Geometry: final body of the model. Coordinates: model frame, mm. A direction names the side the tool comes from. Round coordinates to 2 decimals unless told otherwise and drop trailing zeros. Loops run counter-clockwise (first coordinate to the right, second up) from the corner with the lowest first, then second, coordinate; pieces in that order, holes last. Notation, with made-up numbers: (-32.75, -10) - (-14.75, -10) arc R19 ccw to (-14.75, 13) - close; hole circle Ø11 at (-21, 42). An arc over 180 degrees is marked (long way). Answer as a JSON object with one key per item and string values. Group by question number.
Item 1: Section C-C (z = 24.5). Count the separate pieces of the cut face and the enclosed holes in it, plus the area to 3 significant figures.
Item 2: Section D-D (x = 21). Return the cut outline in (y, z), plus the area to 3 significant figures.
Item 3: Section A-A (z = 7). Return the cut outline in (x, y).
Item 4: Reachability of faces 4 (the face through (37, 65, 5.25)), 5 (the face through (69, 75, 15)) from +Z, -Z, +X, -X, +Y, -Y: full face, straight path, thin tool, end or side. Return the list, or none.
Item 5: First-contact query: pin 1 (17.5 mm diameter, centred on x = 108.5, y = 36, fed in from +Z); pin 2 (1.7 mm diameter, centred on x = 129.5, y = 67, fed in from +Z); pin 3 (6 mm diameter, centred on x = 19, y = 33.5, fed in from +Z). Flat tips, straight axial feed; report the tip coordinate or a pass-through.
Item 6: Line query: line 1 (X direction, y = 37.5, z = 2.15); line 2 (Y direction, x = 105, z = 12.75); line 3 (Y direction, x = 106, z = 27.5). Output: solid intervals per line, ascending.
Item 7: Draft query along X for faces 1 (the face through (140, 37, 15)), 2 (the face through (69, 0, 15)), 3 (the face through (130, 8, 10)). Return one class per face: released by +X, released by -X, zero draft, split by the parting line, or undercut.
Item 8: Section B-B (x = 105). Return the cut outline in (y, z), plus the area to 3 significant figures.
```python
from build123d import *

# Parameters (mm, degrees)
ESQUISSE1_W                  = 140
ESQUISSE1_H                  = 75
BOSS_EXTRU_1_DEPTH           = 30
ESQUISSE2_R                  = 31
ENL_V_MAT_EXTRU_1_DEPTH      = 25
ENL_V_MAT_EXTRU_2_DEPTH      = 161.779351908
ENL_V_MAT_EXTRU_2_DEPTH_BACK = 161.779351908
ESQUISSE3_R                  = 3.4
BOSS_EXTRU_2_START           = 0.25
ESQUISSE4_R                  = 31
ESQUISSE4_R_2                = 27.01
BOSS_EXTRU_2_DEPTH           = 0.25
BOSS_EXTRU_3_START           = 7.9
ESQUISSE5_R                  = 7.99
ESQUISSE5_R_2                = 3.4
BOSS_EXTRU_3_DEPTH           = 7.9
ESQUISSE6_R                  = 1.65
ENL_V_MAT_EXTRU_3_DEPTH      = 20


with BuildPart() as part:
    # Esquisse1 → Boss.-Extru.1 (new body)
    with BuildSketch(Plane.XY):
        with Locations((70, 37.5)):
            Rectangle(ESQUISSE1_W, ESQUISSE1_H)
    extrude(amount=BOSS_EXTRU_1_DEPTH)

    # Esquisse2 → Enlèv. mat.-Extru.1 (cut)
    with BuildSketch(Plane.XY.offset(30)):
        with Locations((35, 37.5)):
            Circle(ESQUISSE2_R)
        with Locations(Location((105, 37.5, 0), (0, 0, 180))):
            Circle(ESQUISSE2_R)
    extrude(amount=-ENL_V_MAT_EXTRU_1_DEPTH, mode=Mode.SUBTRACT)

    # Esquisse3 → Enlèv. mat.-Extru.2 (cut, two sides: drawn at the far end of the back side and taken through both)
    with BuildSketch(Plane.XY.offset(5).offset(-ENL_V_MAT_EXTRU_2_DEPTH_BACK)):
        with Locations((35, 37.5)):
            Circle(ESQUISSE3_R)
        with Locations(Location((105, 37.5, 0), (0, 0, 180))):
            Circle(ESQUISSE3_R)
    extrude(amount=ENL_V_MAT_EXTRU_2_DEPTH + ENL_V_MAT_EXTRU_2_DEPTH_BACK, mode=Mode.SUBTRACT)

    # Esquisse4 → Boss.-Extru.2 (add)
    # profile 1 of 2: a face of its own
    with BuildSketch(Plane.XY.offset(5).offset(BOSS_EXTRU_2_START)):
        with Locations((35, 37.5)):
            Circle(ESQUISSE4_R)
        with Locations((35, 37.5)):
            Circle(ESQUISSE4_R_2, mode=Mode.SUBTRACT)
    # profile 2 of 2: a face of its own
    with BuildSketch(Plane.XY.offset(5).offset(BOSS_EXTRU_2_START)):
        with Locations(Location((105, 37.5, 0), (0, 0, 180))):
            Circle(ESQUISSE4_R)
        with Locations(Location((105, 37.5, 0), (0, 0, 180))):
            Circle(ESQUISSE4_R_2, mode=Mode.SUBTRACT)
    extrude(amount=-BOSS_EXTRU_2_DEPTH)

    # Esquisse5 → Boss.-Extru.3 (add)
    # profile 1 of 2: a face of its own
    with BuildSketch(Plane.XY.offset(5).offset(BOSS_EXTRU_3_START)):
        with Locations((35, 37.5)):
            Circle(ESQUISSE5_R)
        with Locations((35, 37.5)):
            Circle(ESQUISSE5_R_2, mode=Mode.SUBTRACT)
    # profile 2 of 2: a face of its own
    with BuildSketch(Plane.XY.offset(5).offset(BOSS_EXTRU_3_START)):
        with Locations(Location((105, 37.5, 0), (0, 0, 180))):
            Circle(ESQUISSE5_R)
        with Locations((105, 37.5)):
            Circle(ESQUISSE5_R_2, mode=Mode.SUBTRACT)
    extrude(amount=-BOSS_EXTRU_3_DEPTH)

    # Esquisse6 → Enlèv. mat.-Extru.3 (cut)
    with BuildSketch(Plane.XY.offset(30)):
        with Locations((60, 67.5)):
            Circle(ESQUISSE6_R)
        with Locations((10, 67.5)):
            Circle(ESQUISSE6_R)
        with Locations(Location((10, 7.5, 0), (0, 0, 180))):
            Circle(ESQUISSE6_R)
        with Locations(Location((60, 7.5, 0), (0, 0, 180))):
            Circle(ESQUISSE6_R)
        with Locations((80, 7.5)):
            Circle(ESQUISSE6_R)
        with Locations((130, 7.5)):
            Circle(ESQUISSE6_R)
        with Locations(Location((130, 67.5, 0), (0, 0, 180))):
            Circle(ESQUISSE6_R)
        with Locations(Location((80, 67.5, 0), (0, 0, 180))):
            Circle(ESQUISSE6_R)
    extrude(amount=-ENL_V_MAT_EXTRU_3_DEPTH, mode=Mode.SUBTRACT)


solid = part.part
```
Values:
{
 "1": {"separate pieces": "1", "enclosed holes": "10", "area": "4,390 mm^2"},
 "2": {"outline": "(0, 0) - (75, 0) - (75, 30) - (65.16, 30) - (65.16, 5.25) - (60.6, 5.25) - (60.6, 5) - (14.4, 5) - (14.4, 5.25) - (9.84, 5.25) - (9.84, 30) - (0, 30) - close", "area": "869 mm^2"},
 "3": {"outline": "(0, 0) - (140, 0) - (140, 75) - (0, 75) - close; circle Ø15.98 at (35, 37.5); circle Ø15.98 at (105, 37.5); hole circle Ø62 at (35, 37.5); hole circle Ø6.8 at (35, 37.5); hole circle Ø62 at (105, 37.5); hole circle Ø6.8 at (105, 37.5)"},
 "4": {"face 4": "+Z", "face 5": "+Z, -Z, +X, -X, +Y"},
 "5": {"pin 1": "stops at z = 12.9", "pin 2": "stops at z = 10", "pin 3": "stops at z = 5"},
 "6": {"line 1": "x = 0 to 31.6, 38.4 to 101.6, 108.4 to 140", "line 2": "y = 0 to 6.5, 29.51 to 34.1, 40.9 to 45.49, 68.5 to 75", "line 3": "y = 0 to 6.52, 68.48 to 75"},
 "7": {"face 1": "released by +X", "face 2": "zero draft", "face 3": "undercut"},
 "8": {"outline": "(0, 0) - (34.1, 0) - (34.1, 12.9) - (29.51, 12.9) - (29.51, 5) - (10.49, 5) - (10.49, 5.25) - (6.5, 5.25) - (6.5, 30) - (0, 30) - close; (40.9, 0) - (75, 0) - (75, 30) - (68.5, 30) - (68.5, 5.25) - (64.51, 5.25) - (64.51, 5) - (45.49, 5) - (45.49, 12.9) - (40.9, 12.9) - close", "area": "741 mm^2"}
}
